from build123d import *

# Parameters (mm, degrees)
EXTRUDE_1_DEPTH = 8
SKETCH_2_R      = 1.5
EXTRUDE_2_DEPTH = 6
M3X0_5_1_D      = 2.5
M3X0_5_1_DEPTH  = 6.5
M3X0_5_1_TIP    = 0.751075774


with BuildPart() as part:
    # 草图1 → 拉伸1 (new body)
    with BuildSketch(Plane.XY):
        Polygon((1.443375673, -2.5), (2.886751346, 0), (1.443375673, 2.5), (-1.443375673, 2.5), (-2.886751346, 0), (-1.443375673, -2.5), align=None)
    extrude(amount=EXTRUDE_1_DEPTH)

    # 草图2 → 拉伸2 (add)
    with BuildSketch(Plane.XY.offset(8)):
        Circle(SKETCH_2_R)
    extrude(amount=EXTRUDE_2_DEPTH)

    # M3x0.5 螺纹孔1
    with Locations(Plane(origin=(0, 0, 0), x_dir=(-1, 0, 0), z_dir=(0, 0, -1))):
        with Locations((0, 0)):
            Hole(M3X0_5_1_D / 2, depth=M3X0_5_1_DEPTH)
            with Locations((0, 0, -(M3X0_5_1_DEPTH + M3X0_5_1_TIP / 2))):  # 118° drill point
                Cone(0, M3X0_5_1_D / 2, M3X0_5_1_TIP, mode=Mode.SUBTRACT)


solid = part.part
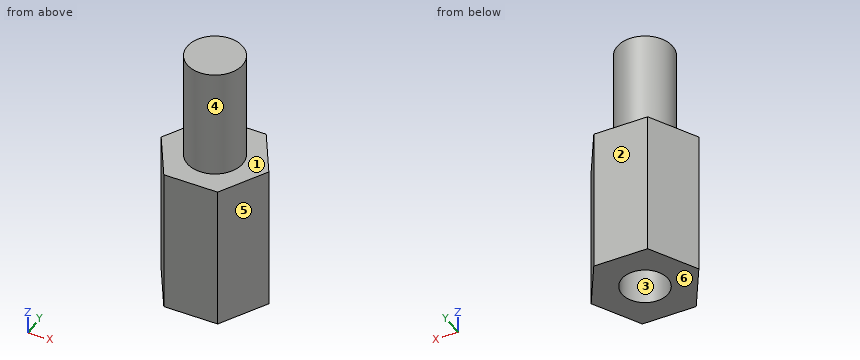
Design review of the part built by this model. Coordinates are the model's own, in mm. Face numbers are marked on the shaded views. A direction names the side the tool comes from. Coordinates: 2 decimals unless noted, no trailing zeros. Loops run counter-clockwise (first coordinate to the right, second up) from the corner with the lowest first, then second, coordinate; pieces in that order, holes last.
Item 1: For the marked faces 1 and 2, list the 3-axis set-ups (+Z, -Z, +X, -X, +Y, -Y) from which the entire face can be reached by the end or side of a thin tool; tool diameter is ignored.
Completed:
face 1: +Z
face 2: +Z, -Z, +X, -X, +Y
Item 2: Add section B-B (x = 2.2). Write out the cut boundary in (y, z), and give its area (3 significant figures).
Completed:
outline: (-1.19, 0) - (1.19, 0) - (1.19, 8) - (-1.19, 8) - close
area: 19.0 mm2
Item 3: Wall thickness on L1, parallel to Y at x = 0, z = 2.5; L2, parallel to Y at x = -0.55, z = 1; L3, parallel to Z at x = 0.4, y = 1.6: over which ranges is each line inside the solid? List them lowest first.
Completed:
L1: y = -2.5 to -1.25, 1.25 to 2.5
L2: y = -2.5 to -1.12, 1.12 to 2.5
L3: z = 0 to 8
Item 4: Draft analysis for pull direction X (two halves, no side actions). For the marked faces 3, 4, 5 and 6, state which applies: pulls with the +X half, pulls with the -X half, needs draft (parallel to the pull), parting line crosses it, or undercut.
Completed:
face 3: undercut
face 4: parting line crosses it
face 5: pulls with the +X half
face 6: needs draft
Item 5: Add section A-A (x = -1.8). Write out the cut boundary in (y, z).
Completed:
outline: (-1.88, 0) - (1.88, 0) - (1.88, 8) - (-1.88, 8) - close
Item 6: Clearance check with flat-ended pins moving along their axes: pin 1 (1 mm diameter, centred on x = -1.5, z = 12, fed in from -Y); pin 2 (1 mm diameter, centred on x = 0.5, y = 0, fed in from -Z). State where each tip first meets the part, or that it passes through.
Completed:
pin 1: stops at y = -1.12
pin 2: stops at z = 6.65
